```python
from build123d import *

# Parameters (mm, degrees)
SKETCH1_W           = 12.5
SKETCH1_H           = 10
BOSS_EXTRUDE1_DEPTH = 10
SKETCH2_W           = 10
SKETCH2_H           = 10
BOSS_EXTRUDE2_DEPTH = 5
SKETCH3_R           = 4
BOSS_EXTRUDE3_DEPTH = 17
SKETCH4_W           = 4
SKETCH4_H           = 10
CUT_EXTRUDE1_DEPTH  = 11
SKETCH5_W           = 9.5
SKETCH5_H           = 10
BOSS_EXTRUDE4_DEPTH = 12.5
SKETCH6_W           = 5
SKETCH6_H           = 10
BOSS_EXTRUDE5_DEPTH = 30
SKETCH7_R           = 1.75
CUT_EXTRUDE2_DEPTH  = 23.5
SKETCH8_W           = 30
SKETCH8_H           = 5
CUT_EXTRUDE4_DEPTH  = 10
SKETCH10_W          = 9.5
SKETCH10_H          = 10
CUT_EXTRUDE6_DEPTH  = 3.49
SKETCH11_W          = 9.5
SKETCH11_H          = 10
BOSS_EXTRUDE6_DEPTH = 3.9
SKETCH12_W          = 4
SKETCH12_H          = 10
BOSS_EXTRUDE7_DEPTH = 20
SKETCH13_W          = 20
SKETCH13_H          = 0.09
CUT_EXTRUDE7_DEPTH  = 28
SKETCH14_R          = 1.75
CUT_EXTRUDE8_DEPTH  = 23.91


with BuildPart() as part:
    # Sketch1 → Boss-Extrude1 (new body)
    with BuildSketch(Plane.XY):
        with Locations((6.25, 5)):
            Rectangle(SKETCH1_W, SKETCH1_H)
    extrude(amount=BOSS_EXTRUDE1_DEPTH)

    # Sketch2 → Boss-Extrude2 (add)
    with BuildSketch(Plane.ZY):
        with Locations((5, 5)):
            Rectangle(SKETCH2_W, SKETCH2_H)
    extrude(amount=BOSS_EXTRUDE2_DEPTH)

    # Sketch3 → Boss-Extrude3 (add)
    with BuildSketch(Plane(origin=(0, 10, 0), x_dir=(1, 0, 0), z_dir=(0, 1, 0))):
        with Locations((3.75, -5)):
            Circle(SKETCH3_R)
    extrude(amount=BOSS_EXTRUDE3_DEPTH)

    # Sketch4 → Cut-Extrude1 (cut, through all)
    with BuildSketch(Plane(origin=(0, 10, 0), x_dir=(1, 0, 0), z_dir=(0, 1, 0))):
        with Locations((10.5, -5)):
            Rectangle(SKETCH4_W, SKETCH4_H)
        with Locations((-3, -5)):
            Rectangle(SKETCH4_W, SKETCH4_H)
    extrude(amount=-CUT_EXTRUDE1_DEPTH, mode=Mode.SUBTRACT)

    # Sketch5 → Boss-Extrude4 (add)
    with BuildSketch(Plane.XY.offset(10)):
        with Locations((3.75, 5)):
            Rectangle(SKETCH5_W, SKETCH5_H)
    extrude(amount=BOSS_EXTRUDE4_DEPTH)

    # Sketch6 → Boss-Extrude5 (add)
    with BuildSketch(Plane(origin=(8.5, 0, 0), x_dir=(0, 0, -1), z_dir=(1, 0, 0))):
        with Locations((-20, 5)):
            Rectangle(SKETCH6_W, SKETCH6_H)
    extrude(amount=BOSS_EXTRUDE5_DEPTH)

    # Sketch7 → Cut-Extrude2 (cut, through all)
    with BuildSketch(Plane.XY.offset(22.5)):
        with Locations((22.5, 5)):
            Circle(SKETCH7_R)
        with Locations((33.5, 5)):
            Circle(SKETCH7_R)
    extrude(amount=-CUT_EXTRUDE2_DEPTH, mode=Mode.SUBTRACT)

    # Sketch8 → Cut-Extrude4 (cut)
    with BuildSketch(Plane(origin=(0, 10, 0), x_dir=(1, 0, 0), z_dir=(0, 1, 0))):
        with Locations((23.5, -20)):
            Rectangle(SKETCH8_W, SKETCH8_H)
    extrude(amount=-CUT_EXTRUDE4_DEPTH, mode=Mode.SUBTRACT)

    # Sketch10 → Cut-Extrude6 (cut)
    with BuildSketch(Plane.XY.offset(22.5)):
        with Locations((3.75, 5)):
            Rectangle(SKETCH10_W, SKETCH10_H)
    extrude(amount=-CUT_EXTRUDE6_DEPTH, mode=Mode.SUBTRACT)

    # Sketch11 → Boss-Extrude6 (add)
    with BuildSketch(Plane.XY.offset(19.01)):
        with Locations((3.75, 5)):
            Rectangle(SKETCH11_W, SKETCH11_H)
    extrude(amount=BOSS_EXTRUDE6_DEPTH)

    # Sketch12 → Boss-Extrude7 (add)
    with BuildSketch(Plane(origin=(8.5, 0, 0), x_dir=(0, 0, -1), z_dir=(1, 0, 0))):
        with Locations((-20.91, 5)):
            Rectangle(SKETCH12_W, SKETCH12_H)
    extrude(amount=BOSS_EXTRUDE7_DEPTH)

    # Sketch13 → Cut-Extrude7 (cut, through all)
    with BuildSketch(Plane(origin=(0, 0, 0), x_dir=(-1, 0, 0), z_dir=(0, -1, 0))):
        with Locations((-18.5, -18.955)):
            Rectangle(SKETCH13_W, SKETCH13_H)
    extrude(amount=-CUT_EXTRUDE7_DEPTH, mode=Mode.SUBTRACT)

    # Sketch14 → Cut-Extrude8 (cut, through all)
    with BuildSketch(Plane.XY.offset(22.91)):
        with Locations((16, 5)):
            Circle(SKETCH14_R)
        with Locations((24.5, 5)):
            Circle(SKETCH14_R)
    extrude(amount=-CUT_EXTRUDE8_DEPTH, mode=Mode.SUBTRACT)


solid = part.part
```
Geometry check sheet. Reference: the model listing, model coordinates, mm. A direction names the side the tool comes from. Coordinates: 2 decimals unless noted, no trailing zeros. Order: outer loops, then holes, each group sorted by start corner. A loop starts at its lowest first (then second) coordinate and runs counter-clockwise, first axis right, second up. Notation, with made-up numbers: M 82.25,-26.75 L 111.25,-26.75 A29 cw 111.25,7.25 Z; hole C 24,25.25 d11. An arc over 180 degrees is marked long. Answer as a JSON object with one key per item and string values.
Q1. Scan lines: line 1 (Y direction, x = 24.5, z = 21.75); line 2 (Z direction, x = 10.25, y = 1.5); line 3 (X direction, y = 2.5, z = 11). Record each from-to range of solid material in increasing order.
Results are:
{"line 1": "y = 0 to 3.25, 6.75 to 10", "line 2": "z = 19 to 22.91", "line 3": "x = -1 to 8.5"}
Q2. Tool access check on faces 4 (the flat face through (7, 0, 14)), 5 (the flat face through (8.5, 5, 9)). Record the directions out of +Z, -Z, +X, -X, +Y, -Y that give a thin tool (end or side, any length) a straight path to the whole face; none if there is none.
Results are:
{"face 4": "+Z, -Z, +X, -X, -Y", "face 5": "-Z, +X, +Y, -Y"}
Q3. Cross-section at A-A on x = 16. Record the cut outline in (y, z).
Results are:
{"outline": "M 0,19 L 3.25,19 L 3.25,22.91 L 0,22.91 Z; M 6.75,19 L 10,19 L 10,22.91 L 6.75,22.91 Z"}
Q4. Depth check by flat-ended pin: pin 1 Ø5.5 at (x, y) = (24.5, 5) entering from -Z; pin 2 Ø3 at (y, z) = (7, 10) entering from +X. Enter the tip coordinate at first touch or a pass-through.
Results are:
{"pin 1": "stops at z = 19", "pin 2": "stops at x = 8.5"}
Q5. Cross-section at C-C on z = 6.25. Record the cut outline in (x, y), and give its area (3 significant figures).
Results are:
{"outline": "M -1,0 L 8.5,0 L 8.5,10 L 7.55,10 L 7.55,27 L -0.05,27 L -0.05,10 L -1,10 Z", "area": "224 mm²"}
Q6. Release check for a two-part mould opening along X. For faces 1 (the cylindrical face through (2.883, 18.381, 8.905)), 2 (the cylindrical face through (16.81, 3.45, 20.98)), 3 (the flat face through (-1, 5, 11)) record: released by +X, released by -X, zero draft, split by the parting line, or undercut.
Results are:
{"face 1": "split by the parting line", "face 2": "undercut", "face 3": "released by -X"}
Q7. Cross-section at B-B on y = 5. Record the cut outline in (x, z).
Results are:
{"outline": "M -1,0 L 8.5,0 L 8.5,19 L 14.25,19 L 14.25,22.91 L -1,22.91 Z; M 17.75,19 L 22.75,19 L 22.75,22.91 L 17.75,22.91 Z; M 26.25,19 L 28.5,19 L 28.5,22.91 L 26.25,22.91 Z"}
Q8. Cross-section at D-D on y = 15. Record the cut outline in (x, z).
Results are:
{"outline": "C 3.75,5 d8"}
